Check sheet for the modelled part. Datum: model origin and axes. Units: mm. Face numbers are marked on the shaded views. Round coordinates to 2 decimals unless told otherwise and drop trailing zeros. Loops run counter-clockwise (first coordinate to the right, second up) from the corner with the lowest first, then second, coordinate; pieces in that order, holes last. Notation, with made-up numbers: M 84,27 L 106,27 A19 ccw 106,40 Z; hole C 33,-39.75 d2. An arc over 180 degrees is marked long. Write item = value, one per line. Start each with the question number.
(1) Cross-section at D-D on y = -19. Record the boundary of the cut face in (x, z).
(2) Go/stop test with flat-tipped pins: P1, Ø4, axis at x = 18.5, y = -73, coming from the -Z side; P2, Ø2, axis at x = 24.5, y = -16, coming from the -Z side. Record where each tip stops, or that it passes through.
(3) Mould release check, pull along Y, two halves, no side actions. Record for the marked faces 1 and 2: pulls with the +Y half, pulls with the -Y half, needs draft (parallel to the pull), parting line crosses it, or undercut.
(4) Scan lines: L1, parallel to Y at x = 5, z = -2.05; L2, parallel to Y at x = 5, z = -1.7; L3, parallel to Y at x = 25, z = -2.25. Record each from-to range of solid material in increasing order. Write a range as from..to.
(5) Cross-section at C-C on y = -2.5. Record the boundary of the cut face in (x, z).
(6) Cross-section at A-A on x = 17.5. Record the boundary of the cut face in (y, z), plus the area to 3 significant figures.
(7) Cross-section at B-B on z = -1.1. Record the boundary of the cut face in (x, y).
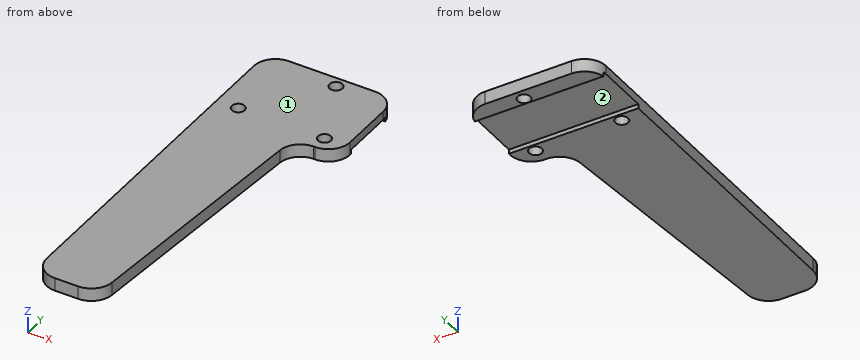
from build123d import *

# Parameters (mm, degrees)
CROQUIS1_R              = 1.5
SALIENTE_EXTRUIR1_DEPTH = 3
CROQUIS2_W              = 30
CROQUIS2_H              = 13
CORTAR_EXTRUIR2_DEPTH   = 1


with BuildPart() as part:
    # Croquis1 → Saliente-Extruir1 (new body)
    with BuildSketch(Plane.XY):
        with BuildLine():
            Line((0, -5), (0, -83))
            ThreePointArc((0, -83), (1.464466094, -86.535533906), (5, -88))
            Line((5, -88), (10.367132634, -88))
            ThreePointArc((10.367132634, -88), (13.765451273, -86.667619177), (15.352628079, -83.380572171))
            Line((15.352628079, -83.380572171), (19.647371921, -27.119427829))
            ThreePointArc((19.647371921, -27.119427829), (21.234548727, -23.832380823), (24.632867366, -22.5))
            Line((24.632867366, -22.5), (25, -22.5))
            ThreePointArc((25, -22.5), (28.535533906, -21.035533906), (30, -17.5))
            Line((30, -17.5), (30, -5))
            ThreePointArc((30, -5), (28.535533906, -1.464466094), (25, 0))
            Line((25, 0), (5, 0))
            ThreePointArc((5, 0), (1.464466094, -1.464466094), (0, -5))
        make_face()
        with Locations((17.5, -2.5)):
            Circle(CROQUIS1_R, mode=Mode.SUBTRACT)
        with Locations((5, -19)):
            Circle(CROQUIS1_R, mode=Mode.SUBTRACT)
        with Locations((25, -19)):
            Circle(CROQUIS1_R, mode=Mode.SUBTRACT)
    extrude(amount=-SALIENTE_EXTRUIR1_DEPTH)

    # Croquis2 → Cortar-Extruir2 (cut)
    with BuildSketch(Plane(origin=(0, 0, -3), x_dir=(-1, 0, 0), z_dir=(0, 0, -1))):
        with Locations((-15, -10.6)):
            Rectangle(CROQUIS2_W, CROQUIS2_H)
    extrude(amount=-CORTAR_EXTRUIR2_DEPTH, mode=Mode.SUBTRACT)


solid = part.part
Result:
q1.outline = M 0,-3 L 3.5,-3 L 3.5,0 L 0,0 Z; M 6.5,-3 L 23.5,-3 L 23.5,0 L 6.5,0 Z; M 26.5,-3 L 29.77,-3 L 29.77,0 L 26.5,0 Z
q2.P1 = through
q2.P2 = -2
q3.face_1 = needs draft
q3.face_2 = undercut
q4.L1 = -88..-20.5, -17.5..-17.1, -4.1..0
q4.L2 = -88..-20.5, -17.5..0
q4.L3 = -22.5..-20.5, -17.5..-17.1, -4.1..0
q5.outline = M 0.67,-3 L 16,-3 L 16,0 L 0.67,0 Z; M 19,-3 L 29.33,-3 L 29.33,0 L 19,0 Z
q6.outline = M -55.25,-3 L -17.1,-3 L -17.1,-2 L -4.1,-2 L -4.1,-3 L -4,-3 L -4,0 L -55.25,0 Z; M -1,-3 L 0,-3 L 0,0 L -1,0 Z
q6.area = 144 mm^2
q7.outline = M 0,-83 A5 ccw 5,-88 L 10.37,-88 A5 ccw 15.35,-83.38 L 19.65,-27.12 A5 cw 24.63,-22.5 L 25,-22.5 A5 ccw 30,-17.5 L 30,-5 A5 ccw 25,0 L 5,0 A5 ccw 0,-5 Z; hole C 5,-19 d3; hole C 17.5,-2.5 d3; hole C 25,-19 d3
